```python
from build123d import *

# Parameters (mm, degrees)
F2_R      = 6.5
F3_DEPTH  = 30
F4_W      = 107.489927
F4_H      = 49.906041
F5_DEPTH  = 15
F3_FACE_R = 6.5
F6_DEPTH  = 15
F7_SIZE   = 5


with BuildPart() as f1:
    # F0 (on Right) → F1 (revolve)
    with BuildSketch(Plane.YZ):
        with BuildLine():
            Line((0, -25.4), (0, 25.4))
            ThreePointArc((0, 25.4), (-25.4, 0), (0, -25.4))
        make_face()
    revolve(axis=Axis((0, 0, 0), (0, 0, -1)))

    # F2 (on Top) → F3 (cut)
    with BuildSketch(Plane.XY):
        Circle(F2_R)
    extrude(amount=-F3_DEPTH, mode=Mode.SUBTRACT)

    # F4 (on Front) → F5 (cut, symmetric)
    with BuildSketch(Plane.XZ):
        with Locations((11.955445, -46.953021)):
            Rectangle(F4_W, F4_H)
    extrude(amount=F5_DEPTH, both=True, mode=Mode.SUBTRACT)

    # F3_face (on face) → F6 (cut)
    with BuildSketch(Plane(origin=(0, 0, 0), x_dir=(1, 0, 0), z_dir=(0, 0, -1))):
        Circle(F3_FACE_R)
    extrude(amount=-F6_DEPTH, mode=Mode.SUBTRACT)

    # F7
    f7_edges = [f1.edges().sort_by_distance(p)[0] for p in [
        (-6.5, 0, 15),
    ]]
    chamfer(f7_edges, length=F7_SIZE)


solid = f1.part
```
The listing builds one solid part. Answer for the finished solid, in the listing's coordinates (mm). Coordinates: 2 decimals unless noted, no trailing zeros. Loops run counter-clockwise (first coordinate to the right, second up) from the corner with the lowest first, then second, coordinate; pieces in that order, holes last. Notation, with made-up numbers: (17, 24) -> (28, 24) arc R35 ccw to (28, 58) -> close; hole circle Ø3 at (8.5, 61.5). An arc over 180 degrees is marked (long way). Return JSON: item names as keys, results as strings. Group by question number.
(1) A cutting plane is placed at D-D on z = 21. Write down the section's boundary in (x, y), and give its area (3 significant figures).
(2) A cutting plane is placed at A-A on x = 0. Write down the section's boundary in (y, z).
(3) A cutting plane is placed at C-C on z = 6.5. Write down the section's boundary in (x, y), and give its area (3 significant figures).
(4) Determine the mould class of faces 1 (the flat face through (-6, -3, -22)), 2 (the flat face through (0, 0, 15)) for opening direction X: released by +X, released by -X, zero draft, split by the parting line, or undercut.
(5) Given pin 1 Ø2.5 at (x, y) = (0.5, 0.5) entering from -Z; pin 2 Ø4 at (y, z) = (7, -15.5) entering from +X; pin 3 Ø1.5 at (y, z) = (-5.5, -10.5) entering from -X, each flat-ended and moving along its own axis, determine where each tip first touches the part or whether it passes through.
(6) Find the intervals of material crossed by probe 1 along Y at (x, z) = (0, 2); probe 2 along X at (y, z) = (-6, -12.5); probe 3 along X at (y, z) = (-21.5, -0.5), in increasing order. Write a range as from..to.
The answers:
{
 "1": {"outline": "circle Ø28.58 at (0, 0)", "area": "641 mm^2"},
 "2": {"outline": "(-12.69, -22) -> (-6.5, -22) -> (-6.5, 10) -> (-1.5, 15) -> (1.5, 15) -> (6.5, 10) -> (6.5, -22) -> (12.69, -22) arc R25.4 ccw (long way) to start"},
 "3": {"outline": "circle Ø49.11 at (0, 0); hole circle Ø13 at (0, 0)", "area": "1,760 mm^2"},
 "4": {"face 1": "zero draft", "face 2": "undercut"},
 "5": {"pin 1": "stops at z = 14.54", "pin 2": "stops at x = 20.49", "pin 3": "stops at x = -22.84"},
 "6": {"probe 1": "y = -25.32..-6.5, 6.5..25.32", "probe 2": "x = -21.28..-2.5, 2.5..21.28", "probe 3": "x = -13.52..13.52"}
}
